```python
from build123d import *

# Parameters (mm, degrees)
SKETCH1_R             = 50
BOSS_EXTRUDE1_DEPTH   = 5
CAVITY1_START         = 1
CAVITY1_OUTLINE_R     = 4.45
CAVITY1_OUTLINE_R_2   = 3.45
CAVITY1_OUTLINE_R_3   = 2.9
CAVITY1_DEPTH         = 2.65
CAVITY1_START_2       = 2
CAVITY1_2_OUTLINE_R   = 4.45
CAVITY1_2_OUTLINE_R_2 = 3.45
CAVITY1_2_OUTLINE_R_3 = 2.9
CAVITY1_2_OUTLINE_R_4 = 1.5
CAVITY1_2_DEPTH       = 1.65
CAVITY1_START_3       = 3.65
CAVITY1_3_OUTLINE_R   = 4.25
CAVITY1_3_OUTLINE_R_2 = 3
CAVITY1_3_DEPTH       = 1.35
CUT_EXTRUDE4_DEPTH    = 4
CUT_EXTRUDE5_START    = -10
SKETCH4_R             = 50
SKETCH4_W             = 40
SKETCH4_H             = 40
CUT_EXTRUDE5_DEPTH    = 10


# Read off the part's stored shape, not the designer's step: Cavity1
with BuildPart() as part:
    # Sketch1 → Boss-Extrude1 (new body)
    with BuildSketch(Plane(origin=(0, 0, 0), x_dir=(1, 0, 0), z_dir=(0, 1, 0))):
        with Locations(Location((0, 0, 0), (0, 0, 270))):
            Circle(SKETCH1_R)
    extrude(amount=BOSS_EXTRUDE1_DEPTH)

    # Cavity1 outline → Cavity1 (cut)
    # profile 1 of 2: a face of its own
    with BuildSketch(Plane(origin=(0, 0, 0), x_dir=(1, 0, 0), z_dir=(0, 1, 0)).offset(CAVITY1_START)):
        with BuildLine():
            Line((-3.736481777, -6.923723208), (-2, -16.771800738))
            ThreePointArc((-2, -16.771800738), (0, -18.45), (2, -16.771800738))
            Line((2, -16.771800738), (3.736481777, -6.923723208))
            ThreePointArc((3.736481777, -6.923723208), (4.670003178, -4.670003178), (6.923723208, -3.736481777))
            Line((6.923723208, -3.736481777), (16.771800738, -2))
            ThreePointArc((16.771800738, -2), (18.45, 0), (16.771800738, 2))
            Line((16.771800738, 2), (6.923723208, 3.736481777))
            ThreePointArc((6.923723208, 3.736481777), (4.670003178, 4.670003178), (3.736481777, 6.923723208))
            Line((3.736481777, 6.923723208), (2, 16.771800738))
            ThreePointArc((2, 16.771800738), (0, 18.45), (-2, 16.771800738))
            Line((-2, 16.771800738), (-3.736481777, 6.923723208))
            ThreePointArc((-3.736481777, 6.923723208), (-4.670003178, 4.670003178), (-6.923723208, 3.736481777))
            Line((-6.923723208, 3.736481777), (-16.771800738, 2))
            ThreePointArc((-16.771800738, 2), (-18.45, 0), (-16.771800738, -2))
            Line((-16.771800738, -2), (-6.923723208, -3.736481777))
            ThreePointArc((-6.923723208, -3.736481777), (-4.670003178, -4.670003178), (-3.736481777, -6.923723208))
        make_face()
        Circle(CAVITY1_OUTLINE_R, mode=Mode.SUBTRACT)
    # profile 2 of 2: a face of its own
    with BuildSketch(Plane(origin=(0, 0, 0), x_dir=(1, 0, 0), z_dir=(0, 1, 0)).offset(CAVITY1_START)):
        Circle(CAVITY1_OUTLINE_R_2)
        Circle(CAVITY1_OUTLINE_R_3, mode=Mode.SUBTRACT)
    extrude(amount=CAVITY1_DEPTH, mode=Mode.SUBTRACT)

    # Cavity1 2 outline → Cavity1 2 (cut)
    # profile 1 of 2: a face of its own
    with BuildSketch(Plane(origin=(0, 0, 0), x_dir=(1, 0, 0), z_dir=(0, 1, 0)).offset(CAVITY1_START_2)):
        Circle(CAVITY1_2_OUTLINE_R)
        Circle(CAVITY1_2_OUTLINE_R_2, mode=Mode.SUBTRACT)
    # profile 2 of 2: a face of its own
    with BuildSketch(Plane(origin=(0, 0, 0), x_dir=(1, 0, 0), z_dir=(0, 1, 0)).offset(CAVITY1_START_2)):
        Circle(CAVITY1_2_OUTLINE_R_3)
        Circle(CAVITY1_2_OUTLINE_R_4, mode=Mode.SUBTRACT)
    extrude(amount=CAVITY1_2_DEPTH, mode=Mode.SUBTRACT)

    # Cavity1 3 outline → Cavity1 3 (cut)
    with BuildSketch(Plane(origin=(0, 0, 0), x_dir=(1, 0, 0), z_dir=(0, 1, 0)).offset(CAVITY1_START_3)):
        Circle(CAVITY1_3_OUTLINE_R)
        Circle(CAVITY1_3_OUTLINE_R_2, mode=Mode.SUBTRACT)
    extrude(amount=CAVITY1_3_DEPTH, mode=Mode.SUBTRACT)

    # Sketch2 → Cut-Extrude4 (cut)
    with BuildSketch(Plane(origin=(0, 1, 0), x_dir=(1, 0, 0), z_dir=(0, 1, 0))):
        with BuildLine():
            Line((-6.957554218, 4.136687101), (-16.841260009, 2.393923101))
            ThreePointArc((-16.841260009, 2.393923101), (-18.85, 0), (-16.841260009, -2.393923101))
            Line((-16.841260009, -2.393923101), (-6.957554218, -4.136687101))
            ThreePointArc((-6.957554218, -4.136687101), (-4.952845891, -4.952845891), (-4.136687101, -6.957554218))
            Line((-4.136687101, -6.957554218), (-2.393923101, -16.841260009))
            ThreePointArc((-2.393923101, -16.841260009), (0, -18.85), (2.393923101, -16.841260009))
            Line((2.393923101, -16.841260009), (4.136687101, -6.957554218))
            ThreePointArc((4.136687101, -6.957554218), (4.952845891, -4.952845891), (6.957554218, -4.136687101))
            Line((6.957554218, -4.136687101), (16.841260009, -2.393923101))
            ThreePointArc((16.841260009, -2.393923101), (18.85, 0), (16.841260009, 2.393923101))
            Line((16.841260009, 2.393923101), (6.957554218, 4.136687101))
            ThreePointArc((6.957554218, 4.136687101), (4.952845891, 4.952845891), (4.136687101, 6.957554218))
            Line((4.136687101, 6.957554218), (2.393923101, 16.841260009))
            ThreePointArc((2.393923101, 16.841260009), (0, 18.85), (-2.393923101, 16.841260009))
            Line((-2.393923101, 16.841260009), (-4.136687101, 6.957554218))
            ThreePointArc((-4.136687101, 6.957554218), (-4.952845891, 4.952845891), (-6.957554218, 4.136687101))
        make_face()
    extrude(amount=CUT_EXTRUDE4_DEPTH, mode=Mode.SUBTRACT)

    # Sketch4 → Cut-Extrude5 (cut)
    with BuildSketch(Plane(origin=(0, 5, 0), x_dir=(1, 0, 0), z_dir=(0, 1, 0)).offset(CUT_EXTRUDE5_START)):
        Circle(SKETCH4_R)
        Rectangle(SKETCH4_W, SKETCH4_H, mode=Mode.SUBTRACT)
    extrude(amount=CUT_EXTRUDE5_DEPTH, mode=Mode.SUBTRACT)


solid = part.part
```
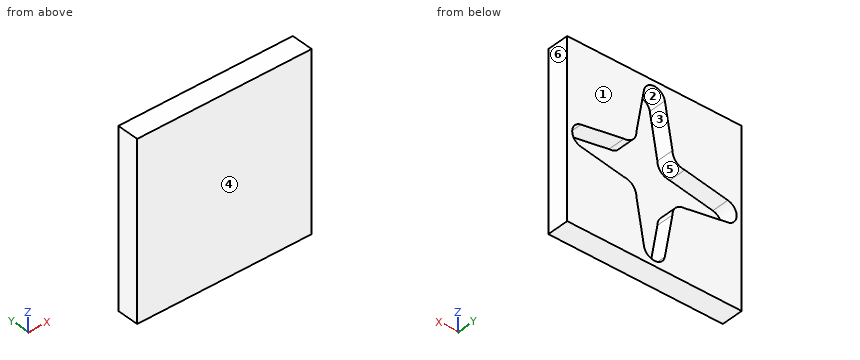
Geometry: final body of the model. Coordinates: model frame, mm. Face numbers are marked on the shaded views. A direction names the side the tool comes from. Coordinates: 2 decimals unless noted, no trailing zeros. Order: outer loops, then holes, each group sorted by start corner. A loop starts at its lowest first (then second) coordinate and runs counter-clockwise, first axis right, second up. Notation, with made-up numbers: M 22,57.25 L 76,57.25 A26 cw 76,73.25 Z; hole C 64,22 d11. An arc over 180 degrees is marked long. Answer in a Markdown table with one row per item. Add a question column.
Q1. Section query A-A on y = 2.1. Return the cut outline in (x, z), and give its area (3 significant figures).
Q2. Reachability of the marked faces 1 and 2 from +Z, -Z, +X, -X, +Y, -Y: full face, straight path, thin tool, end or side. Return the list, or none.
Q3. Mould query, pull axis X, two halves, no side actions, for the marked faces 3, 4, 5 and 6. Classes: released by +X, released by -X, zero draft, split by the parting line, or undercut.
Q4. Section query B-B on x = 15. Return the cut outline in (y, z), and give its area (3 significant figures).
Q5. Line query: L1, parallel to X at y = 1.8, z = 7; L2, parallel to Y at x = 3.5, z = -10; L3, parallel to Z at x = 12, y = 1.2. Output: solid intervals per line, ascending.
Q6. Section query C-C on z = 18. Return the cut outline in (x, y).
Completed:
| question | item | result |
|---|---|---|
| 1 | outline | M -20,-20 L 20,-20 L 20,20 L -20,20 Z; hole M -16.84,-2.39 L -6.96,-4.14 A2.79 cw -4.14,-6.96 L -2.39,-16.84 A2.43 ccw 2.39,-16.84 L 4.14,-6.96 A2.79 cw 6.96,-4.14 L 16.84,-2.39 A2.43 ccw 16.84,2.39 L 6.96,4.14 A2.79 cw 4.14,6.96 L 2.39,16.84 A2.43 ccw -2.39,16.84 L -4.14,6.96 A2.79 cw -6.96,4.14 L -16.84,2.39 A2.43 ccw Z |
| 1 | area | 1,140 mm2 |
| 2 | face 1 | +Z, -Z, +X, -X, +Y |
| 2 | face 2 | +Y |
| 3 | face 3 | undercut |
| 3 | face 4 | zero draft |
| 3 | face 5 | undercut |
| 3 | face 6 | released by +X |
| 4 | outline | M 0,-20 L 5,-20 L 5,-2.72 L 1,-2.72 L 1,2.72 L 5,2.72 L 5,20 L 0,20 Z |
| 4 | area | 178 mm2 |
| 5 | L1 | x = -20 to -4.13, 4.13 to 20 |
| 5 | L2 | y = 0 to 1 |
| 5 | L3 | z = -20 to -3.25, 3.25 to 20 |
| 6 | outline | M -20,0 L 20,0 L 20,5 L 1.85,5 L 1.85,1 L -1.85,1 L -1.85,5 L -20,5 Z |
